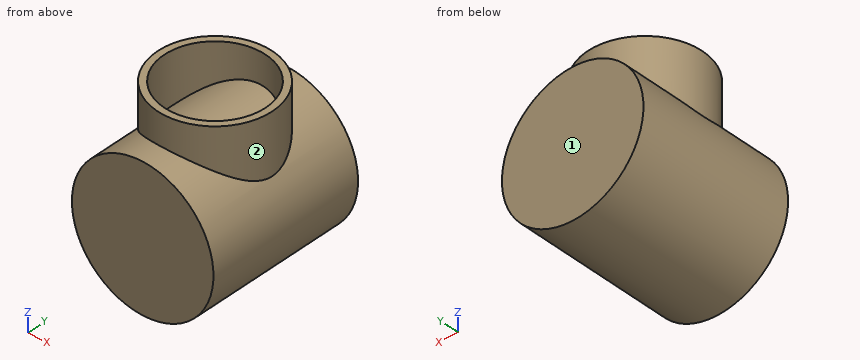
```python
from build123d import *

# Parameters (mm, degrees)
SKETCH1_R                = 21
BOSS_EXTRUDE1_DEPTH      = 47.8
BOSS_EXTRUDE2_REACH      = 74.985
BOSS_EXTRUDE2_END_RADIUS = 21
SKETCH3_R                = 17
SKETCH3_R_2              = 15


with BuildPart() as part:
    # Sketch1 → Boss-Extrude1 (new body)
    with BuildSketch(Plane(origin=(0, 0, 0), x_dir=(1, 0, 0), z_dir=(0, 1, 0))):
        with Locations(Location((0, 0, 0), (0, 0, 90))):
            Circle(SKETCH1_R)
    extrude(amount=BOSS_EXTRUDE1_DEPTH)

    # Boss-Extrude2: up to this cylinder (the profile starts outside it)
    boss_extrude2_end = Plane(origin=(0, 23.9, 0), z_dir=(0, -1, 0)) * Cylinder(BOSS_EXTRUDE2_END_RADIUS, 192.97, mode=Mode.PRIVATE)
    # Sketch3 → Boss-Extrude2 (add, up to the surface)
    with BuildSketch(Plane.XY.offset(30), mode=Mode.PRIVATE) as boss_extrude2_sk1:
        with Locations((0, 23.9)):
            Circle(SKETCH3_R)
        with Locations((0, 23.9)):
            Circle(SKETCH3_R_2, mode=Mode.SUBTRACT)
    boss_extrude2_tool1 = extrude(boss_extrude2_sk1.sketch, amount=-BOSS_EXTRUDE2_REACH, mode=Mode.PRIVATE) - boss_extrude2_end
    add(boss_extrude2_tool1.solids().sort_by_distance((-16.519167, 23.9, 30))[0])


solid = part.part
```
Input: part model. Units: mm. Frame: model coordinates. Face numbers are marked on the shaded views. A direction names the side the tool comes from. Round coordinates to 2 decimals unless told otherwise and drop trailing zeros. Loops run counter-clockwise (first coordinate to the right, second up) from the corner with the lowest first, then second, coordinate; pieces in that order, holes last. Notation, with made-up numbers: (79, 26) -> (112, 26) arc R35 ccw to (112, 65) -> close; hole circle Ø8 at (54, 29). An arc over 180 degrees is marked (long way). One line per item, written item: value.
(1) Section C-C (z = 24.5). Return the cut outline in (x, y), plus the area to 3 significant figures.
Geometry check:
outline: circle Ø34 at (0, 23.9); hole circle Ø30 at (0, 23.9)
area: 201 mm2
(2) Material intervals for line 1 (X direction, y = 23.9, z = 21.5); line 2 (X direction, y = 23.9, z = 18); line 3 (X direction, y = 3.5, z = 0), sorted ascending. Write a range as [from, to].
Geometry check:
line 1: [-17, -15], [15, 17]
line 2: [-17, -15], [-10.82, 10.82], [15, 17]
line 3: [-21, 21]
(3) Section D-D (x = -6). Return the cut outline in (y, z).
Geometry check:
outline: (0, -20.12) -> (47.8, -20.12) -> (47.8, 20.12) -> (39.81, 20.12) -> (39.81, 30) -> (37.65, 30) -> (37.65, 20.12) -> (10.15, 20.12) -> (10.15, 30) -> (7.99, 30) -> (7.99, 20.12) -> (0, 20.12) -> close
(4) Set-up query: the marked faces 1 and 2. Return all of +Z, -Z, +X, -X, +Y, -Y with unobstructed straight access to the full face (end or side cutting, diameter ignored); none if empty.
Geometry check:
face 1: +Z, -Z, +X, -X, +Y
face 2: +Z
(5) Section A-A (x = 0). Return the cut outline in (y, z), plus the area to 3 significant figures.
Geometry check:
outline: (0, -21) -> (47.8, -21) -> (47.8, 21) -> (40.9, 21) -> (40.9, 30) -> (38.9, 30) -> (38.9, 21) -> (8.9, 21) -> (8.9, 30) -> (6.9, 30) -> (6.9, 21) -> (0, 21) -> close
area: 2,040 mm2
(6) Pin query (flat end, axial travel): pin 1 (3 mm diameter, centred on y = 9, z = 10.5, fed in from -X); pin 2 (6 mm diameter, centred on y = 17, z = 7, fed in from +X); pin 3 (12 mm diameter, centred on x = -14.5, y = 22.5, fed in from +Z); pin 4 (4 mm diameter, centred on y = 40, z = 16, fed in from -X). Return the tip coordinate at first contact, or that it passes through.
Geometry check:
pin 1: x = -18.97
pin 2: x = 20.62
pin 3: z = 30
pin 4: x = -15.65
(7) Section B-B (y = 23.9). Return the cut outline in (x, z).
Geometry check:
outline: (-17, 12.33) arc R21 ccw (long way) to (17, 12.33) -> (17, 30) -> (15, 30) -> (15, 14.7) arc R21 ccw to (-15, 14.7) -> (-15, 30) -> (-17, 30) -> close
